Work out the finished part from the listing and answer in its coordinate system (mm). Face numbers are marked on the shaded views. Round coordinates to 2 decimals unless told otherwise and drop trailing zeros. Loops run counter-clockwise (first coordinate to the right, second up) from the corner with the lowest first, then second, coordinate; pieces in that order, holes last. Notation, with made-up numbers: (35, -25.75) -> (43, -25.75) arc R27 ccw to (43, 5.25) -> close; hole circle Ø5 at (-16, 72). An arc over 180 degrees is marked (long way). Use CSV: the item, a comma, the result in double quotes. Start each with the question number.
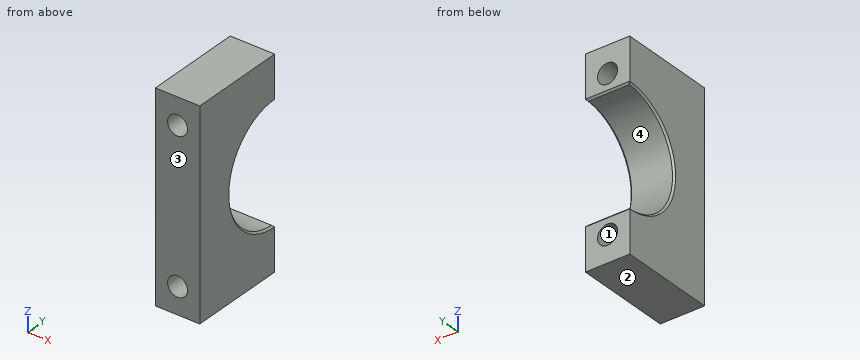
from build123d import *

# Parameters (mm, degrees)
BOSS_EXTRUDE1_DEPTH                           = 15.875
BOSS_EXTRUDE2_DEPTH                           = 15.875
CBORE_FOR_1_4_SOCKET_HEAD_CAP_SCREW1_AT_COUNT = 2
CBORE_FOR_1_4_SOCKET_HEAD_CAP_SCREW1_AT_PITCH = 53.975
MOVE_FACE1_BY                                 = 0.127
MOVE_FACE1_2_BY                               = 0.127
MOVE_START                                    = 28.575
MOVE_FACE2_OUTLINE_W                          = 15.875
MOVE_FACE2_OUTLINE_H                          = 73.025
MOVE_FACE2_OUTLINE_R                          = 5.55625
MOVE_FACE2_DEPTH                              = 6.35
MOVE_START_2                                  = 22.225
MOVE_FACE2_2_OUTLINE_R                        = 5.55625
MOVE_FACE2_2_OUTLINE_R_2                      = 3.57124
MOVE_FACE2_2_DEPTH                            = 6.35


with BuildPart() as part:
    # Sketch1 → Boss-Extrude1 (new body)
    with BuildSketch(Plane(origin=(0, 0, 0), x_dir=(0, 0, -1), z_dir=(1, 0, 0))):
        with BuildLine():
            Line((36.5125, 0), (20.6375, 0))
            ThreePointArc((20.6375, 0), (0, -20.6375), (-20.6375, 0))
            Line((-20.6375, 0), (-36.5125, 0))
            Line((-36.5125, 0), (-36.5125, -34.925))
            Line((-36.5125, -34.925), (36.5125, -34.925))
            Line((36.5125, -34.925), (36.5125, 0))
        make_face()
    extrude(amount=BOSS_EXTRUDE1_DEPTH)


with BuildPart() as body_2:
    # Sketch1<3> → Boss-Extrude2 (new body)
    with BuildSketch(Plane(origin=(0, 0, 0), x_dir=(0, 0, -1), z_dir=(1, 0, 0))):
        with BuildLine():
            ThreePointArc((-20.6375, 0), (0, 20.6375), (20.6375, 0))
            Line((20.6375, 0), (36.5125, 0))
            Line((36.5125, 0), (36.5125, 34.925))
            Line((36.5125, 34.925), (-36.5125, 34.925))
            Line((-36.5125, 34.925), (-36.5125, 0))
            Line((-36.5125, 0), (-20.6375, 0))
        make_face()
    extrude(amount=BOSS_EXTRUDE2_DEPTH)


with BuildPart() as cbore_for_1_4_socket_head_cap_screw1_tool:
    # Sketch4 → CBORE for 1/4 Socket Head Cap Screw1 (revolve)
    with BuildSketch(Plane(origin=(7.9375, 34.925, 26.9875), x_dir=(0, 0, 1), z_dir=(1, 0, 0))):
        Polygon((0, 0), (0, 69.85), (3.57124, 69.85), (3.57124, 6.35), (5.55625, 6.35), (5.55625, 0.635), (6.19125, 0), align=None)
    cbore_for_1_4_socket_head_cap_screw1 = revolve(axis=Axis((7.9375, 41.275, 26.9875), (0, -1, 0)))


with BuildPart() as part_1:
    add(part.part)

    # CBORE for 1/4 Socket Head Cap Screw1: cut by cbore_for_1_4_socket_head_cap_screw1_tool
    add(cbore_for_1_4_socket_head_cap_screw1_tool.part, mode=Mode.SUBTRACT)


with BuildPart() as body_2_1:
    add(body_2.part)

    # CBORE for 1/4 Socket Head Cap Screw1: cut by cbore_for_1_4_socket_head_cap_screw1_tool
    add(cbore_for_1_4_socket_head_cap_screw1_tool.part, mode=Mode.SUBTRACT)


with BuildPart() as cbore_for_1_4_socket_head_cap_screw1_at_tool:
    # CBORE for 1/4 Socket Head Cap Screw1 at: CBORE for 1/4 Socket Head Cap Screw1 ×2
    with Locations(*[(0, 0, -i * CBORE_FOR_1_4_SOCKET_HEAD_CAP_SCREW1_AT_PITCH) for i in range(1, CBORE_FOR_1_4_SOCKET_HEAD_CAP_SCREW1_AT_COUNT)]):
        add(cbore_for_1_4_socket_head_cap_screw1)


with BuildPart() as part_2:
    add(part_1.part)

    # CBORE for 1/4 Socket Head Cap Screw1 at: cut by cbore_for_1_4_socket_head_cap_screw1_at_tool
    add(cbore_for_1_4_socket_head_cap_screw1_at_tool.part, mode=Mode.SUBTRACT)

    # Move Face1 2: a curved face moved inward by 0.127
    add(Solid.thicken(part_2.faces().sort_by_distance((7.9375, -20.6375, 0))[0], -MOVE_FACE1_2_BY), mode=Mode.SUBTRACT)

    # Chamfer1
    # the kernel refuses this chamfer: 0.635 mm, written as the material it takes off along each edge
    with BuildSketch(Plane(origin=(0, 0, 0), x_dir=(0, 0.07868977926472538, -0.9968991516895122), z_dir=(0, 0.9968991516895122, 0.07868977926472538))) as chamfer1_piece_1:
        with BuildLine():
            Line((21.417460512, 0.017960512), (20.746539488, -0.652960512))
            Line((20.746539488, -0.652960512), (20.733839488, -0.652960512))
            ThreePointArc((20.733839488, -0.652960512), (20.7518, -0.326480256), (20.7518, 0))
            Line((20.7518, 0), (20.7645, 0.0127))
            ThreePointArc((20.7645, 0.0127), (21.090980256, 0.0127), (21.417460512, 0.030660512))
            Line((21.417460512, 0.030660512), (21.417460512, 0.017960512))
        make_face()
    revolve(axis=Axis((0, 0, 0), (-1, 0, 0)), revolution_arc=189.026516368, mode=Mode.SUBTRACT)
    with BuildSketch(Plane(origin=(-1.610111621, 0, -20.7645), x_dir=(0, 0, -1), z_dir=(1, 0, 0))) as chamfer1_piece_2:
        with BuildLine():
            Line((0.643801601, 0.017692029), (-0.027368853, -0.633849299))
            Line((-0.027368853, -0.633849299), (-0.040063261, -0.633472445))
            ThreePointArc((-0.040063261, -0.633472445), (-0.015119867, -0.316902726), (-0.0127, 0))
            Line((-0.0127, 0), (0, 0.0127))
            ThreePointArc((0, 0.0127), (0.3219008, 0.0127), (0.643801601, 0.030392029))
            Line((0.643801601, 0.030392029), (0.643801601, 0.017692029))
        make_face()
    extrude(amount=19.095223242, mode=Mode.SUBTRACT)
    with BuildSketch(Plane(origin=(-1.610111621, 0, 20.7645), x_dir=(0, -0.9998899044534173, -0.01483842889716635), z_dir=(1, 0, 0))) as chamfer1_piece_3:
        with BuildLine():
            Line((0.634185626, 0.017960512), (-0.027243086, -0.643468199))
            Line((-0.027243086, -0.643468199), (-0.039941687, -0.643279751))
            ThreePointArc((-0.039941687, -0.643279751), (-0.017475104, -0.321676913), (-0.012698602, 0.000188448))
            Line((-0.012698602, 0.000188448), (0.000188448, 0.012698602))
            ThreePointArc((0.000188448, 0.012698602), (0.317092192, 0.010415864), (0.633997178, 0.030659114))
            Line((0.633997178, 0.030659114), (0.634185626, 0.017960512))
        make_face()
    extrude(amount=19.095223242, mode=Mode.SUBTRACT)
    with BuildSketch(Plane(origin=(15.875, 0, 0), x_dir=(0, 0.0786897792647254, -0.9968991516895122), z_dir=(0, 0.9968991516895122, 0.0786897792647254))) as chamfer1_piece_4:
        with BuildLine():
            Line((20.746539488, 0.652960512), (21.417460512, -0.017960512))
            Line((21.417460512, -0.017960512), (21.417460512, -0.030660512))
            ThreePointArc((21.417460512, -0.030660512), (21.090980256, -0.0127), (20.7645, -0.0127))
            Line((20.7645, -0.0127), (20.7518, 0))
            ThreePointArc((20.7518, 0), (20.7518, 0.326480256), (20.733839488, 0.652960512))
            Line((20.733839488, 0.652960512), (20.746539488, 0.652960512))
        make_face()
    revolve(axis=Axis((15.875, 0, 0), (-1, 0, 0)), revolution_arc=189.026516368, mode=Mode.SUBTRACT)


with BuildPart() as body_2_2:
    add(body_2_1.part)

    # CBORE for 1/4 Socket Head Cap Screw1 at: cut by cbore_for_1_4_socket_head_cap_screw1_at_tool
    add(cbore_for_1_4_socket_head_cap_screw1_at_tool.part, mode=Mode.SUBTRACT)

    # Move Face1: a curved face moved inward by 0.127
    add(Solid.thicken(body_2_2.faces().sort_by_distance((7.9375, 20.6375, 0))[0], -MOVE_FACE1_BY), mode=Mode.SUBTRACT)

    # Move Face2: read off the stored shape, not the designer's step
    # Move Face2 outline → Move Face2 (cut)
    with BuildSketch(Plane(origin=(0, 0, 0), x_dir=(1, 0, 0), z_dir=(0, 1, 0)).offset(MOVE_START)):
        with Locations((7.9375, 0)):
            Rectangle(MOVE_FACE2_OUTLINE_W, MOVE_FACE2_OUTLINE_H)
        with Locations((7.9375, -26.9875)):
            Circle(MOVE_FACE2_OUTLINE_R, mode=Mode.SUBTRACT)
        with Locations((7.9375, 26.9875)):
            Circle(MOVE_FACE2_OUTLINE_R, mode=Mode.SUBTRACT)
    extrude(amount=MOVE_FACE2_DEPTH, mode=Mode.SUBTRACT)

    # Move Face2 2 outline → Move Face2 2 (cut)
    # profile 1 of 2: a face of its own
    with BuildSketch(Plane(origin=(0, 0, 0), x_dir=(1, 0, 0), z_dir=(0, 1, 0)).offset(MOVE_START_2)):
        with Locations((7.9375, 26.9875)):
            Circle(MOVE_FACE2_2_OUTLINE_R)
        with Locations((7.9375, 26.9875)):
            Circle(MOVE_FACE2_2_OUTLINE_R_2, mode=Mode.SUBTRACT)
    # profile 2 of 2: a face of its own
    with BuildSketch(Plane(origin=(0, 0, 0), x_dir=(1, 0, 0), z_dir=(0, 1, 0)).offset(MOVE_START_2)):
        with Locations((7.9375, -26.9875)):
            Circle(MOVE_FACE2_2_OUTLINE_R)
        with Locations((7.9375, -26.9875)):
            Circle(MOVE_FACE2_2_OUTLINE_R_2, mode=Mode.SUBTRACT)
    extrude(amount=MOVE_FACE2_2_DEPTH, mode=Mode.SUBTRACT)

    # Move Face2 3: loft between two sections, ruled curve by curve
    move_face2_3_from = [
        Edge.make_three_point_arc((7.9375, 27.94, -21.43125), (13.49375, 27.94, -26.9875), (7.9375, 27.94, -32.54375)),
        Edge.make_three_point_arc((7.9375, 27.94, -32.54375), (2.38125, 27.94, -26.9875), (7.9375, 27.94, -21.43125)),
    ]
    move_face2_3_to = [
        Edge.make_three_point_arc((7.9375, 28.575, -20.79625), (14.12875, 28.575, -26.9875), (7.9375, 28.575, -33.17875)),
        Edge.make_three_point_arc((7.9375, 28.575, -33.17875), (1.74625, 28.575, -26.9875), (7.9375, 28.575, -20.79625)),
    ]
    move_face2_3 = Solid(Shell([*[Face.make_surface_from_curves(move_face2_3_from[k], move_face2_3_to[k]) for k in range(2)], Face(Wire(move_face2_3_from)), Face(Wire(move_face2_3_to))]))
    add(move_face2_3, mode=Mode.SUBTRACT)

    # Move Face2 4: loft between two sections, ruled curve by curve
    move_face2_4_from = [
        Edge.make_three_point_arc((7.9375, 27.94, 32.54375), (13.49375, 27.94, 26.9875), (7.9375, 27.94, 21.43125)),
        Edge.make_three_point_arc((7.9375, 27.94, 21.43125), (2.38125, 27.94, 26.9875), (7.9375, 27.94, 32.54375)),
    ]
    move_face2_4_to = [
        Edge.make_three_point_arc((7.9375, 28.575, 33.17875), (14.12875, 28.575, 26.9875), (7.9375, 28.575, 20.79625)),
        Edge.make_three_point_arc((7.9375, 28.575, 20.79625), (1.74625, 28.575, 26.9875), (7.9375, 28.575, 33.17875)),
    ]
    move_face2_4 = Solid(Shell([*[Face.make_surface_from_curves(move_face2_4_from[k], move_face2_4_to[k]) for k in range(2)], Face(Wire(move_face2_4_from)), Face(Wire(move_face2_4_to))]))
    add(move_face2_4, mode=Mode.SUBTRACT)

    # Chamfer2
    # the kernel refuses this chamfer: 0.635 mm, written as the material it takes off along each edge
    with BuildSketch(Plane(origin=(0, 0, 0), x_dir=(0, -0.0786897792647251, 0.9968991516895122), z_dir=(0, -0.9968991516895122, -0.0786897792647251))) as chamfer2_piece_1:
        with BuildLine():
            Line((21.417460512, 0.017960512), (20.746539488, -0.652960512))
            Line((20.746539488, -0.652960512), (20.733839488, -0.652960512))
            ThreePointArc((20.733839488, -0.652960512), (20.7518, -0.326480256), (20.7518, 0))
            Line((20.7518, 0), (20.7645, 0.0127))
            ThreePointArc((20.7645, 0.0127), (21.090980256, 0.0127), (21.417460512, 0.030660512))
            Line((21.417460512, 0.030660512), (21.417460512, 0.017960512))
        make_face()
    revolve(axis=Axis((0, 0, 0), (-1, 0, 0)), revolution_arc=189.026516368, mode=Mode.SUBTRACT)
    with BuildSketch(Plane(origin=(-1.610111621, 0, 20.7645), x_dir=(0, 0, 1), z_dir=(1, 0, 0))) as chamfer2_piece_2:
        with BuildLine():
            Line((0.643801601, 0.017692029), (-0.027368853, -0.633849299))
            Line((-0.027368853, -0.633849299), (-0.040063261, -0.633472445))
            ThreePointArc((-0.040063261, -0.633472445), (-0.015119867, -0.316902726), (-0.0127, 0))
            Line((-0.0127, 0), (0, 0.0127))
            ThreePointArc((0, 0.0127), (0.3219008, 0.0127), (0.643801601, 0.030392029))
            Line((0.643801601, 0.030392029), (0.643801601, 0.017692029))
        make_face()
    extrude(amount=19.095223242, mode=Mode.SUBTRACT)
    with BuildSketch(Plane(origin=(-1.610111621, 0, -20.7645), x_dir=(0, 0.9998899044534173, 0.014838428897166573), z_dir=(1, 0, 0))) as chamfer2_piece_3:
        with BuildLine():
            Line((0.634185626, 0.017960512), (-0.027243086, -0.643468199))
            Line((-0.027243086, -0.643468199), (-0.039941687, -0.643279751))
            ThreePointArc((-0.039941687, -0.643279751), (-0.017475104, -0.321676913), (-0.012698602, 0.000188448))
            Line((-0.012698602, 0.000188448), (0.000188448, 0.012698602))
            ThreePointArc((0.000188448, 0.012698602), (0.317092192, 0.010415864), (0.633997178, 0.030659114))
            Line((0.633997178, 0.030659114), (0.634185626, 0.017960512))
        make_face()
    extrude(amount=19.095223242, mode=Mode.SUBTRACT)
    with BuildSketch(Plane(origin=(15.875, 0, 0), x_dir=(0, -0.07868977926472513, 0.9968991516895122), z_dir=(0, -0.9968991516895122, -0.07868977926472513))) as chamfer2_piece_4:
        with BuildLine():
            Line((20.746539488, 0.652960512), (21.417460512, -0.017960512))
            Line((21.417460512, -0.017960512), (21.417460512, -0.030660512))
            ThreePointArc((21.417460512, -0.030660512), (21.090980256, -0.0127), (20.7645, -0.0127))
            Line((20.7645, -0.0127), (20.7518, 0))
            ThreePointArc((20.7518, 0), (20.7518, 0.326480256), (20.733839488, 0.652960512))
            Line((20.733839488, 0.652960512), (20.746539488, 0.652960512))
        make_face()
    revolve(axis=Axis((15.875, 0, 0), (-1, 0, 0)), revolution_arc=189.026516368, mode=Mode.SUBTRACT)


solid = part_2.part
Q1. For a pull along Z with two mould halves and no side action, classify the marked faces 1, 2, 3 and 4 as pulls with the +Z half, pulls with the -Z half, needs draft (parallel to the pull), parting line crosses it, or undercut.
Q2. Section A-A, the plane x = 7 is taken. Write down the section's boundary in (y, z) (1 decimal), and give its area (3 significant figures).
Q3. Straight lines are drawn through the part: line 1 (Z direction, x = 5.5, y = -31.5); line 2 (Z direction, x = 7, y = -8); line 3 (Z direction, x = 11, y = -28). For each, find the intervals that lie inside material, in ascending order. Write a range as from..to.
Q4. Each of these flat-tipped pins is pushed along its axis until it touches: pin 1 (2 mm diameter, centred on x = 5.5, z = -6.5, fed in from +Y); pin 2 (5 mm diameter, centred on x = 7, z = 3.5, fed in from +Y). Where does it stop, or does it pass through?
Q5. Section D-D, the plane y = -16 is taken. Give the number of separate pieces and of enclosed holes in the cut face, and give its area (3 significant figures).
Q6. Section B-B, the plane z = 27 is taken. Write down the section's boundary in (x, y) (3 decimals), and give its area (3 significant figures).
Report:
1,face 1,"undercut"
1,face 2,"pulls with the -Z half"
1,face 3,"needs draft"
1,face 4,"undercut"
2,outline,"(-34.9, -36.5) -> (0, -36.5) -> (0, -30.4) -> (-34.9, -30.4) -> close; (-34.9, -23.5) -> (0, -23.5) -> (0, -21.4) -> (-0.6, -20.8) arc R20.8 cw to (-0.6, 20.8) -> (0, 21.4) -> (0, 23.5) -> (-34.9, 23.5) -> close; (-34.9, 30.4) -> (0, 30.4) -> (0, 36.5) -> (-34.9, 36.5) -> close"
2,area,"1,390 mm²"
3,line 1,"z = -36.51..-29.6, -24.38..24.38, 29.6..36.51"
3,line 2,"z = -36.51..-30.43, -23.54..-19.16, 19.16..23.54, 30.43..36.51"
3,line 3,"z = -36.51..-28.82, -25.15..25.15, 28.82..36.51"
4,pin 1,"stops at y = -19.36"
4,pin 2,"stops at y = -19.88"
5,separate pieces,"2"
5,enclosed holes,"2"
5,area,"658 mm²"
6,outline,"(0, -34.925) -> (4.366, -34.925) -> (4.366, 0) -> (0, 0) -> close; (11.509, -34.925) -> (15.875, -34.925) -> (15.875, 0) -> (11.509, 0) -> close"
6,area,"305 mm²"
